from build123d import *

# Parameters (mm, degrees)
F0_R     = 44.45
F1_DEPTH = 127
F2_DEPTH = 19.05
F3_DEPTH = 107.95
F4_DEPTH = 152.4
F5_DEPTH = 25.4


with BuildPart() as f1:
    # F0 (on Front) → F1 (new body)
    with BuildSketch(Plane.XZ):
        with BuildLine():
            ThreePointArc((186.227747, 226.098122), (127, 266.7), (67.772253, 226.098122))
            ThreePointArc((67.772253, 226.098122), (72.072893, 171.336809), (117.475, 140.418439))
            ThreePointArc((117.475, 140.418439), (127, 139.7), (136.525, 140.418439))
            ThreePointArc((136.525, 140.418439), (175.151259, 161.803065), (190.5, 203.2))
            ThreePointArc((190.5, 203.2), (189.4228, 214.846632), (186.227747, 226.098122))
        make_face()
        with Locations((127, 203.2)):
            Circle(F0_R, mode=Mode.SUBTRACT)
    extrude(amount=F1_DEPTH)

    # F0 (on Front) → F2 (join)
    with BuildSketch(Plane.XZ):
        with BuildLine():
            Line((136.525, 50.8), (254, 50.8))
            Line((254, 50.8), (186.227747, 226.098122))
            ThreePointArc((186.227747, 226.098122), (189.4228, 214.846632), (190.5, 203.2))
            ThreePointArc((190.5, 203.2), (175.151259, 161.803065), (136.525, 140.418439))
            Line((136.525, 140.418439), (136.525, 50.8))
        make_face()
        with BuildLine():
            Line((67.772253, 226.098122), (0, 50.8))
            Line((0, 50.8), (117.475, 50.8))
            Line((117.475, 50.8), (117.475, 140.418439))
            ThreePointArc((117.475, 140.418439), (72.072893, 171.336809), (67.772253, 226.098122))
        make_face()
    extrude(amount=F2_DEPTH)

    # F0 (on Front) → F3 (join)
    with BuildSketch(Plane.XZ):
        with BuildLine():
            Line((117.475, 140.418439), (117.475, 50.8))
            Line((117.475, 50.8), (136.525, 50.8))
            Line((136.525, 50.8), (136.525, 140.418439))
            ThreePointArc((136.525, 140.418439), (127, 139.7), (117.475, 140.418439))
        make_face()
    extrude(amount=F3_DEPTH)

    # F0 (on Front) → F4 (join)
    with BuildSketch(Plane.XZ):
        Polygon((0, 50.8), (0, 0), (254, 0), (254, 50.8), (136.525, 50.8), (117.475, 50.8), align=None)
    extrude(amount=F4_DEPTH)

    # F0 (on Front) → F5 (join)
    with BuildSketch(Plane.XZ):
        with BuildLine():
            ThreePointArc((186.227747, 226.098122), (127, 266.7), (67.772253, 226.098122))
            ThreePointArc((67.772253, 226.098122), (72.072893, 171.336809), (117.475, 140.418439))
            ThreePointArc((117.475, 140.418439), (127, 139.7), (136.525, 140.418439))
            ThreePointArc((136.525, 140.418439), (175.151259, 161.803065), (190.5, 203.2))
            ThreePointArc((190.5, 203.2), (189.4228, 214.846632), (186.227747, 226.098122))
        make_face()
        with Locations((127, 203.2)):
            Circle(F0_R, mode=Mode.SUBTRACT)
        Polygon((0, 50.8), (0, 0), (254, 0), (254, 50.8), (136.525, 50.8), (117.475, 50.8), align=None)
    extrude(amount=F5_DEPTH)


solid = f1.part
For this review, take the finished solid that the model builds, in its own axes (mm). A direction names the side the tool comes from. Round coordinates to 2 decimals unless told otherwise and drop trailing zeros. Order: outer loops, then holes, each group sorted by start corner. A loop starts at its lowest first (then second) coordinate and runs counter-clockwise, first axis right, second up. Notation, with made-up numbers: M 85,-37.75 L 143,-37.75 A21 ccw 143,-29.75 Z; hole C -33,36 d5. An arc over 180 degrees is marked long. Use a Markdown table: item, result. Add a question column.
Item 1: Add section C-C, the plane x = 236. Give the boundary of the cut face in (y, z).
Item 2: To check wall thickness, follow line 1 along Z through (x, y) = (95, -36); line 2 along Z through (x, y) = (127, -61); line 3 along Z through (x, y) = (112.5, -60.5). State the ranges of each line that lie inside material, in increasing order.
Item 3: Tool access review of faces 4 (the cylindrical face through (126.9, -117.3, 139.7)), 5 (the flat face through (136.525, -63, 95)), 6 (the flat face through (71, -19.05, 101)): name each direction out of +Z, -Z, +X, -X, +Y, -Y from which nothing blocks a thin tool from reaching the whole face with its end or side.
Item 4: Mouldability with a two-part tool opening along X and no side actions: class faces 1 (the flat face through (125, -152.4, 26)), 2 (the flat face through (117.475, -63, 96)), 3 (the cylindrical face through (150.9, -62.61, 240.68)) as released by +X, released by -X, zero draft, split by the parting line, or undercut.
Item 5: Insertion check: pin 1 (1.5 mm diameter, centred on y = -122, z = 221, fed in from +X); pin 2 (8 mm diameter, centred on x = 187.5, z = 197, fed in from -Y); pin 3 (15 mm diameter, centred on x = 129.5, z = 91, fed in from -Y); pin 4 (2 mm diameter, centred on x = 49, y = -82, fed in from -Z). Each pin has a flat end and moves straight along its axis. Give the tip position at first contact, or say it passes through.
Item 6: Add section B-B, the plane y = -52.5. Give the boundary of the cut face in (x, z) (3 decimals), then the cut area to 3 significant figures.
Item 7: Add section A-A, the plane x = 127. Give the boundary of the cut face in (y, z), then the cut area to 3 significant figures.
Item 8: Add section D-D, the plane y = -133. Give the boundary of the cut face in (x, z), then the cut area to 3 significant figures.
Geometry results:
| question | item | result |
|---|---|---|
| 1 | outline | M -152.4,0 L 0,0 L 0,97.36 L -19.05,97.36 L -19.05,50.8 L -152.4,50.8 Z |
| 2 | line 1 | z = 0 to 50.8, 148.35 to 172.35, 234.05 to 258.05 |
| 2 | line 2 | z = 0 to 158.75, 247.65 to 266.7 |
| 2 | line 3 | z = 0 to 50.8, 141.38 to 161.18, 245.22 to 265.02 |
| 3 | face 4 | -Y |
| 3 | face 5 | +X, -Y |
| 3 | face 6 | -X, -Y |
| 4 | face 1 | zero draft |
| 4 | face 2 | released by -X |
| 4 | face 3 | undercut |
| 5 | pin 1 | stops at x = 188.17 |
| 5 | pin 2 | stops at y = -127 |
| 5 | pin 3 | stops at y = -107.95 |
| 5 | pin 4 | stops at z = 0 |
| 6 | outline | M 0,0 L 254,0 L 254,50.8 L 136.525,50.8 L 136.525,140.418 A63.5 ccw 190.5,203.2 A63.5 ccw 186.228,226.098 A63.5 ccw long 117.475,140.418 L 117.475,50.8 L 0,50.8 Z; hole C 127,203.2 d88.9 |
| 6 | area | 21,100 mm² |
| 7 | outline | M -152.4,0 L 0,0 L 0,158.75 L -127,158.75 L -127,139.7 L -107.95,139.7 L -107.95,50.8 L -152.4,50.8 Z; M -127,247.65 L 0,247.65 L 0,266.7 L -127,266.7 Z |
| 7 | area | 22,200 mm² |
| 8 | outline | M 0,0 L 254,0 L 254,50.8 L 0,50.8 Z |
| 8 | area | 12,900 mm² |
